Check sheet for the modelled part. Datum: model origin and axes. Units: mm. Coordinates: 2 decimals unless noted, no trailing zeros. Order: outer loops, then holes, each group sorted by start corner. A loop starts at its lowest first (then second) coordinate and runs counter-clockwise, first axis right, second up. Notation, with made-up numbers: M -24.75,-18 L -11.75,-18 A35 ccw -11.75,18 Z; hole C -15.75,89.5 d6. An arc over 180 degrees is marked long. Answer in a Markdown table with one row per item. Add a question column.
from build123d import *

# Parameters (mm, degrees)
F1_DEPTH = 6.35
F2_D     = 5.1054
F3_R     = 3.175


with BuildPart() as f1:
    # F0 (on Front) → F1 (new body)
    with BuildSketch(Plane.XZ):
        Polygon((-30.1625, 0), (0, 0), (30.1625, 0), (30.1625, 33.3375), (0, 33.3375), (-30.1625, 33.3375), align=None)
    extrude(amount=F1_DEPTH)

    # F2 (through all)
    with Locations(Plane(origin=(0, 0, 0), x_dir=(1, 0, 0), z_dir=(0, 1, 0))):
        with Locations((-19.05, -15.875), (19.05, -15.875)):
            Hole(F2_D / 2)

    # F3
    f3_edges = [f1.edges().sort_by_distance(p)[0] for p in [
        (-30.1625, -3.175, 33.3375),
        (30.1625, -3.175, 33.3375),
    ]]
    fillet(f3_edges, radius=F3_R)


solid = f1.part
1. Scan lines: line 1 (X direction, y = -0.75, z = 16); line 2 (X direction, y = -5.5, z = 14.5); line 3 (Z direction, x = -19.05, y = -4.75). Record each from-to range of solid material in increasing order.
2. Section check B-B on y = -4.5. State how many separate pieces and enclosed holes the cut face has, then the cut area to 3 significant figures.
3. Release check for a two-part mould opening along X. For faces 1 (the flat face through (0, -6.35, 17)), 2 (the flat face through (-30.162, -3, 15)), 3 (the cylindrical face through (-17.17, -3.22, 14.15)), 4 (the cylindrical face through (29.26, -3.22, 32.38)) record: released by +X, released by -X, zero draft, split by the parting line, or undercut.
4. Section check A-A on x = -19.05. Enter the section's corners in (y, z).
Result sheet:
| question | item | result |
|---|---|---|
| 1 | line 1 | -30.16 to -21.6, -16.5 to 16.5, 21.6 to 30.16 |
| 1 | line 2 | -30.16 to -21.2, -16.9 to 16.9, 21.2 to 30.16 |
| 1 | line 3 | 0 to 13.32, 18.43 to 33.34 |
| 2 | separate pieces | 1 |
| 2 | enclosed holes | 2 |
| 2 | area | 1,970 mm^2 |
| 3 | face 1 | zero draft |
| 3 | face 2 | released by -X |
| 3 | face 3 | undercut |
| 3 | face 4 | released by +X |
| 4 | outline | M -6.35,0 L 0,0 L 0,13.32 L -6.35,13.32 Z; M -6.35,18.43 L 0,18.43 L 0,33.34 L -6.35,33.34 Z |
